Autodesk Inventor part; units mm, degrees
ref_plane "Piano di lavoro1" through (0, 0, 0) normal (0, 0, 1) x (1, 0, 0)
ref_plane "YZ Plane" through (0, 0, 0) normal (1, 0, 0) x (0, 1, 0)
ref_plane "XZ Plane" through (0, 0, 0) normal (0, 1, 0) x (-1, 0, 0)
ref_plane "Piano di lavoro1" through (0, 0, 0) normal (0, 0, 1) x (1, 0, 0)
sketch "Schizzo1" plane through (0, 0, 0) normal (0, 0, 1) x (1, 0, 0)
  line L0 (42, 54.3) -> (-33, 54.3)
  line L1 (42, 19.3) -> (42, 54.3)
  line L2 (-45, -61) -> (45, -61)
  line L3 (-45, 61) -> (-45, -61)
  line L4 (45, 61) -> (-45, 61)
  circle A0 centre (-40, 57.5) radius 2.5
  circle A1 centre (-40, -42) radius 2.5
  circle A2 centre (41.5, -42) radius 2.5
  circle A3 centre (41.5, 57.5) radius 2.5
  line L5 (45, -61) -> (45, 61)
  line L6 (-45.5, 61.5) -> (-45.5, -61.5)
  line L7 (-45.5, -61.5) -> (45.5, -61.5)
  line L8 (45.5, -61.5) -> (45.5, 61.5)
  line L9 (45.5, 61.5) -> (-45.5, 61.5)
  line L10 (48.5, 64.5) -> (48.5, -64.5)
  line L11 (48.5, -64.5) -> (-48.5, -64.5)
  line L12 (-48.5, -64.5) -> (-48.5, 64.5)
  line L13 (-48.5, 64.5) -> (48.5, 64.5)
  point P0 (0, 0)
  dimension "d0" = 0.5
  dimension "d1" = 3
extrude "Estrusione1" add sketch "Schizzo1" along normal blind 17.25 contours L10 L11 L12 L13
move faces "Sposta1" translate (0, 0, -3) faces at (-47.5, 20.5, 0)
sketch "Schizzo2" plane through (0, 0, 0) normal (0, 0, 1) x (1, 0, 0)
  circle A0 centre (41.5, 57.5) radius 2.5
  circle A1 centre (-40, 57.5) radius 2.5
  circle A2 centre (41.5, -42) radius 2.5
  circle A3 centre (-40, -42) radius 2.5
  line L0 (-45.5, 61.5) -> (45.5, 61.5)
  line L1 (-45.5, 61.5) -> (45.5, 61.5)
  line L2 (45.5, 61.5) -> (45.5, -61.5)
  line L3 (45.5, 61.5) -> (45.5, -61.5)
  line L4 (-45.5, -61.5) -> (-45.5, 61.5)
  line L5 (-45.5, -61.5) -> (-45.5, 61.5)
  line L6 (45.5, -61.5) -> (-45.5, -61.5)
  line L7 (45.5, -61.5) -> (-45.5, -61.5)
  line L8 (45.5, 61.5) -> (37.5, 61.5)
  line L9 (37.5, 61.5) -> (37.5, 55.5)
  line L10 (39.5, 53.5) -> (45.5, 53.5)
  line L11 (45.5, 53.5) -> (45.5, 61.5)
  arc A4 (37.5, 55.5) -> (39.5, 53.5) centre (39.5, 55.5) ccw
  line L12 (-45.5, 61.5) -> (-35.5, 61.5)
  line L13 (-35.5, 61.5) -> (-35.5, 53.5)
  line L14 (-37.5, 51.5) -> (-45.5, 51.5)
  line L15 (-45.5, 51.5) -> (-45.5, 61.5)
  arc A5 (-37.5, 51.5) -> (-35.5, 53.5) centre (-37.5, 53.5) ccw
  line L16 (-45.5, -61.5) -> (-45.5, 61.5)
  line L17 (-45.5, -37.8875) -> (-45.5, -46.8794)
  line L18 (-45.5, -46.496) -> (-38.5282, -46.496)
  line L19 (-36.5282, -44.496) -> (-36.5282, -39.504)
  line L20 (-38.5282, -37.504) -> (-45.5, -37.504)
  arc A6 (-38.5282, -46.496) -> (-36.5282, -44.496) centre (-38.5282, -44.496) ccw
  arc A7 (-36.5282, -39.504) -> (-38.5282, -37.504) centre (-38.5282, -39.504) ccw
  line L21 (45.5, 61.5) -> (45.5, -61.5)
  line L22 (45.5, -45.9102) -> (45.5, -38.0898)
  line L23 (45.5, -38.0898) -> (40.1, -38.0898)
  line L24 (38.1, -40.0898) -> (38.1, -43.9102)
  line L25 (40.1, -45.9102) -> (45.5, -45.9102)
  arc A8 (38.1, -43.9102) -> (40.1, -45.9102) centre (40.1, -43.9102) ccw
  arc A9 (40.1, -38.0898) -> (38.1, -40.0898) centre (40.1, -40.0898) ccw
  point P0 (0, 0)
  point P1 (37.5, 53.5)
  point P2 (-35.5, 51.5)
  point P3 (-36.5282, -42.3835)
  point P4 (-36.5282, -42)
  point P5 (38.1, -38.0898)
  dimension "d7" = 8
  dimension "d8" = 8
  dimension "d9" = 2
  dimension "d10" = 10
  dimension "d11" = 10
  dimension "d12" = 2
  dimension "d13" = 2
  dimension "d14" = 7.4
  dimension "d15" = 2
extrude "Estrusione2" add sketch "Schizzo2" along normal blind 2.5 contours L0 L13 A5 L14 L4 | L0 L2 L10 A4 L9 | L20 A7 L19 A6 L18 L4 | L2 L25 A8 L24 A9 L23
properties part number "_Stampa 3D"
The listing builds one solid part. Answer for the finished solid, in the listing's coordinates (mm). A direction names the side the tool comes from. Round coordinates to 2 decimals unless told otherwise and drop trailing zeros. Write each loop counter-clockwise with the first axis right and the second up, starting at its lowest first coordinate (ties: lowest second). Pieces come first, ordered by that corner, then holes. Notation, with made-up numbers: M 44,-33.5 L 93,-33.5 A6 ccw 93,-25.5 Z; hole C -16,74 d6. An arc over 180 degrees is marked long. Write each question's results on one line, items separated by ' | '. Start each with the question number.
Item 1: For a pull along X with two mould halves and no side action, classify faces 1 (the face through (1, -64.5, 7)), 2 (the face through (44.2, -41.9, 0)), 3 (the face through (48.5, 1, 7)) as pulls with the +X half, pulls with the -X half, needs draft (parallel to the pull), parting line crosses it, or undercut.
Item 2: A cutting plane is placed at C-C on y = 6. Write down the section's boundary in (x, z), and give its area (4 significant figures).
Item 3: For faces 4 (the face through (-42, 55, 2.5)), 5 (the face through (38.1, -42, 1)), 6 (the face through (41.4, 60.2, 0)), determine the directions among +Z, -Z, +X, -X, +Y, -Y from which every point of the face is accessible in a straight line to the end or side of a thin tool.
Item 4: Flat-ended cylindrical pins translate along their axes: pin 1 Ø4 at (x, y) = (42, 58.5) entering from -Z; pin 2 Ø4 at (x, y) = (-40, -42) entering from -Z. Find the tip coordinate at first contact, or state that the pin passes through.
Item 5: A cutting plane is placed at A-A on x = -40. Write down the section's boundary in (y, z), and give its area (3 significant figures).
Item 6: A cutting plane is placed at D-D on x = 23. Write down the section's boundary in (y, z), and give its area (4 significant figures).
Item 7: Straight lines are drawn through the part: L1, parallel to Y at x = 41.5, z = 1.65; L2, parallel to Y at x = -40, z = 0.9; L3, parallel to X at y = 42.5, z = 9. For each, find the intervals that lie inside material, in ascending order. Write a range as [from, to].
Item 8: A cutting plane is placed at B-B on y = 57.5. Write down the section's boundary in (x, z), and give its area (4 significant figures).
Check sheet entries:
1) face 1: needs draft | face 2: undercut | face 3: pulls with the +X half
2) outline: M -48.5,-3 L -45.5,-3 L -45.5,17.25 L -48.5,17.25 Z; M 45.5,-3 L 48.5,-3 L 48.5,17.25 L 45.5,17.25 Z | area: 121.5 mm²
3) face 4: +Z | face 5: +Z, -Z | face 6: -Z
4) pin 1: z = 0 | pin 2: through
5) outline: M -64.5,-3 L -61.5,-3 L -61.5,17.25 L -64.5,17.25 Z; M -46.5,0 L -44.5,0 L -44.5,2.5 L -46.5,2.5 Z; M -39.5,0 L -37.5,0 L -37.5,2.5 L -39.5,2.5 Z; M 51.5,0 L 55,0 L 55,2.5 L 51.5,2.5 Z; M 60,0 L 61.5,0 L 61.5,-3 L 64.5,-3 L 64.5,17.25 L 61.5,17.25 L 61.5,2.5 L 60,2.5 Z | area: 144 mm²
6) outline: M -64.5,-3 L -61.5,-3 L -61.5,17.25 L -64.5,17.25 Z; M 61.5,-3 L 64.5,-3 L 64.5,17.25 L 61.5,17.25 Z | area: 121.5 mm²
7) L1: [-64.5, -61.5], [-45.91, -44.5], [-39.5, -38.09], [53.5, 55], [60, 64.5] | L2: [-64.5, -61.5], [-46.5, -44.5], [-39.5, -37.5], [51.5, 55], [60, 64.5] | L3: [-48.5, -45.5], [45.5, 48.5]
8) outline: M -48.5,-3 L -45.5,-3 L -45.5,0 L -42.5,0 L -42.5,2.5 L -45.5,2.5 L -45.5,17.25 L -48.5,17.25 Z; M -37.5,0 L -35.5,0 L -35.5,2.5 L -37.5,2.5 Z; M 37.5,0 L 39,0 L 39,2.5 L 37.5,2.5 Z; M 44,0 L 45.5,0 L 45.5,-3 L 48.5,-3 L 48.5,17.25 L 45.5,17.25 L 45.5,2.5 L 44,2.5 Z | area: 141.5 mm²
